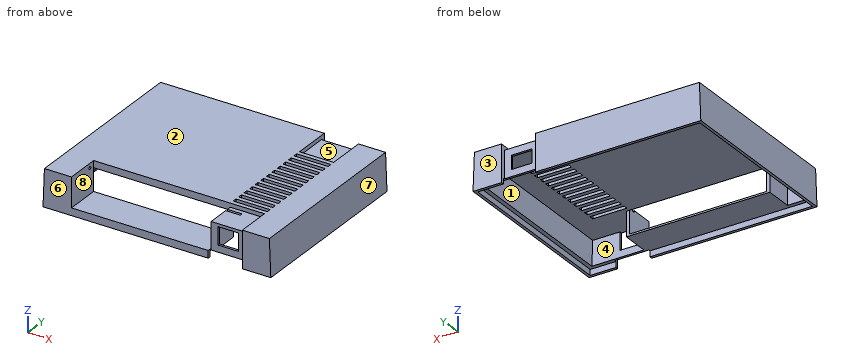
from build123d import *

# Parameters (mm, degrees)
F0_W      = 80
F0_H      = 63
F0_W_2    = 78
F0_H_2    = 61
F1_DEPTH  = 13
F3_DEPTH  = 63
F4_T      = -2.4
F5_DEPTH  = 2
F6_DEPTH  = 1.6
F7_W      = 7.2
F7_H      = 6.2
F8_DEPTH  = 2
F9_W      = 12
F9_H      = 12
F9_H_2    = 10.4
F10_DEPTH = 1.4
F9_H_3    = 1.5
F11_DEPTH = 3
F12_W     = 12
F12_H     = 11.6
F13_DEPTH = 1.6
F14_W     = 7.2
F14_H     = 4.8
F15_DEPTH = 3
F2_W      = 48
F2_H      = 10.4
F16_DEPTH = 12
F17_W     = 1.2
F17_H     = 9.6
F18_DEPTH = 8.6
F19_W     = 9.6
F19_H     = 0.6
F20_DEPTH = 48
F21_D     = 1
F21_DEPTH = 5
F21_TIP   = 0.3004303095
F23_D     = 1
F23_DEPTH = 5
F23_TIP   = 0.3004303095


with BuildPart() as f1:
    # F0 (on Top) → F1 (new body)
    with BuildSketch(Plane.XY):
        Rectangle(F0_W, F0_H)
        Rectangle(F0_W_2, F0_H_2, mode=Mode.SUBTRACT)
        Rectangle(F0_W_2, F0_H_2)
    extrude(amount=F1_DEPTH)

    # F2 (on face) → F3 (cut)
    with BuildSketch(Plane.XZ.offset(31.5)):
        Polygon((-39.5, 13), (-40, 13), (-40, 0), align=None)
        Polygon((39.5, 13), (40, 0), (40, 13), align=None)
    extrude(amount=-F3_DEPTH, mode=Mode.SUBTRACT)

    # F4
    f4_openings = [f1.faces().sort_by_distance(p)[0] for p in [
        (0, 0, 0),
    ]]
    offset(amount=F4_T, openings=f4_openings)

    # F0 (on Top) → F5 (cut)
    with BuildSketch(Plane.XY):
        Rectangle(F0_W_2, F0_H_2)
    extrude(amount=F5_DEPTH, mode=Mode.SUBTRACT)

    # F2 (on face) → F6 (cut)
    with BuildSketch(Plane.XZ.offset(31.5)):
        Polygon((18, 2.6), (18, 0), (30, 0), (30, 13), (18, 13), align=None)
    extrude(amount=-F6_DEPTH, mode=Mode.SUBTRACT)

    # F7 (on face) → F8 (cut)
    with BuildSketch(Plane.XZ.offset(29.9)):
        with Locations((24, 7.5)):
            Rectangle(F7_W, F7_H)
    extrude(amount=-F8_DEPTH, mode=Mode.SUBTRACT)

    # F9 (on face) → F10 (cut)
    with BuildSketch(Plane.XY.offset(13)):
        with Locations((24, 25.5)):
            Rectangle(F9_W, F9_H)
        with Locations((24, -24.7)):
            Rectangle(F9_W, F9_H_2)
    extrude(amount=-F10_DEPTH, mode=Mode.SUBTRACT)

    # F9 (on face) → F11 (cut)
    with BuildSketch(Plane.XY.offset(13)):
        with Locations((24, -17.25)):
            Rectangle(F9_W, F9_H_3)
        with Locations((24, -14.25)):
            Rectangle(F9_W, F9_H_3)
        with Locations((24, -11.25)):
            Rectangle(F9_W, F9_H_3)
        with Locations((24, -8.25)):
            Rectangle(F9_W, F9_H_3)
        with Locations((24, -5.25)):
            Rectangle(F9_W, F9_H_3)
        with Locations((24, 0.75)):
            Rectangle(F9_W, F9_H_3)
        with Locations((24, -2.25)):
            Rectangle(F9_W, F9_H_3)
        with Locations((24, 3.75)):
            Rectangle(F9_W, F9_H_3)
        with Locations((24, 6.75)):
            Rectangle(F9_W, F9_H_3)
        with Locations((24, 9.75)):
            Rectangle(F9_W, F9_H_3)
        with Locations((24, 12.75)):
            Rectangle(F9_W, F9_H_3)
        with Locations((24, 15.75)):
            Rectangle(F9_W, F9_H_3)
        with Locations((24, 18.75)):
            Rectangle(F9_W, F9_H_3)
    extrude(amount=-F11_DEPTH, mode=Mode.SUBTRACT)

    # F12 (on face) → F13 (cut)
    with BuildSketch(Plane(origin=(0, 31.5, 0), x_dir=(-1, 0, 0), z_dir=(0, 1, 0))):
        with Locations((-24, 5.8)):
            Rectangle(F12_W, F12_H)
    extrude(amount=-F13_DEPTH, mode=Mode.SUBTRACT)

    # F14 (on face) → F15 (cut)
    with BuildSketch(Plane(origin=(0, 29.9, 0), x_dir=(-1, 0, 0), z_dir=(0, 1, 0))):
        with Locations((-24, 6.8)):
            Rectangle(F14_W, F14_H)
    extrude(amount=-F15_DEPTH, mode=Mode.SUBTRACT)

    # F2 (on face) → F16 (cut)
    with BuildSketch(Plane.XZ.offset(31.5)):
        with Locations((-6, 7.8)):
            Rectangle(F2_W, F2_H)
    extrude(amount=-F16_DEPTH, mode=Mode.SUBTRACT)

    # F17 (on face) → F18 (join)
    with BuildSketch(Plane(origin=(0, 0, 10.6), x_dir=(1, 0, 0), z_dir=(0, 0, -1))):
        with Locations((18.6, 24.3)):
            Rectangle(F17_W, F17_H)
        with Locations((-30.6, 24.3)):
            Rectangle(F17_W, F17_H)
    extrude(amount=F18_DEPTH)

    # F19 (on face) → F20 (join)
    with BuildSketch(Plane.YZ.offset(-30)):
        with Locations((-24.3, 2.3)):
            Rectangle(F19_W, F19_H)
    extrude(amount=F20_DEPTH)

    # F21 (one way)
    with BuildSketch(Plane.YZ.offset(-30)):
        with Locations((-21.5, 11.4)):
            Circle(F21_D / 2)
    extrude(amount=-F21_DEPTH, mode=Mode.SUBTRACT)
    with Locations(Plane.YZ.offset(-30)):
        with Locations((-21.5, 11.4)):
            with Locations((0, 0, -(F21_DEPTH + F21_TIP / 2))):  # 118° drill point
                Cone(0, F21_D / 2, F21_TIP, mode=Mode.SUBTRACT)

    # F23 (one way)
    with BuildSketch(Plane(origin=(18, 0, 0), x_dir=(0, -1, 0), z_dir=(-1, 0, 0))):
        with Locations((21.5, 11.4)):
            Circle(F23_D / 2)
    extrude(amount=-F23_DEPTH, mode=Mode.SUBTRACT)
    with Locations(Plane(origin=(18, 0, 0), x_dir=(0, -1, 0), z_dir=(-1, 0, 0))):
        with Locations((21.5, 11.4)):
            with Locations((0, 0, -(F23_DEPTH + F23_TIP / 2))):  # 118° drill point
                Cone(0, F23_D / 2, F23_TIP, mode=Mode.SUBTRACT)


solid = f1.part
Input: part model. Units: mm. Frame: model coordinates. Face numbers are marked on the shaded views. A direction names the side the tool comes from. Coordinates: 2 decimals unless noted, no trailing zeros. Loops run counter-clockwise (first coordinate to the right, second up) from the corner with the lowest first, then second, coordinate; pieces in that order, holes last.
(1) Section B-B on z = 7.25. Count the separate pieces of the cut face and the enclosed holes in it, then the cut area to 3 significant figures.
(2) Material intervals for probe 1 along Y at (x, z) = (19.5, 10); probe 2 along Y at (x, z) = (-31, 9.75); probe 3 along Y at (x, z) = (-25.5, 9.5), sorted ascending.
(3) Set-up query: the marked faces 4, 5, 6, 7 and 8. Return all of +Z, -Z, +X, -X, +Y, -Y with unobstructed straight access to the full face (end or side cutting, diameter ignored); none if empty.
(4) Pull-direction query (Y, two-part tool) for the marked faces 1, 2 and 3; classes: released by +Y, released by -Y, zero draft, split by the parting line, or undercut.
(5) First-contact query: pin 1 Ø1.9 at (x, z) = (24, 12) entering from -Y; pin 2 Ø1 at (y, z) = (-8, 10.5) entering from +X; pin 3 Ø2.5 at (y, z) = (-24.5, 5) entering from -X. Flat tips, straight axial feed; report the tip coordinate or a pass-through.
(6) Section C-C on y = 22.5. Return the cut outline in (x, z), then the cut area to 3 significant figures.
(7) Section A-A on x = -17.5. Return the cut outline in (y, z).
Data:
1. separate pieces: 3
1. enclosed holes: 0
1. area: 519 mm2
2. probe 1: y = -29.9 to -29.1, 29.1 to 29.9
2. probe 2: y = -31.5 to -19.5, 29.1 to 31.5
2. probe 3: y = 29.1 to 31.5
3. face 4: -Z
3. face 5: +Z, +Y
3. face 6: +Z, -Z, +X, -X, -Y
3. face 7: +Z, +X, +Y, -Y
3. face 8: +Z, -Y
4. face 1: undercut
4. face 2: zero draft
4. face 3: released by +Y
5. pin 1: stops at y = -29.9
5. pin 2: stops at x = 39.62
5. pin 3: stops at x = -39.86
6. outline: (-40, 0) - (-39, 0) - (-39, 2) - (-37.52, 2) - (-37.19, 10.6) - (37.19, 10.6) - (37.52, 2) - (39, 2) - (39, 0) - (40, 0) - (39.5, 13) - (30, 13) - (30, 11.6) - (18, 11.6) - (18, 13) - (-39.5, 13) - close
6. area: 218 mm2
7. outline: (-31.5, 0) - (-30.5, 0) - (-30.5, 2) - (-19.5, 2) - (-19.5, 2.6) - (-31.5, 2.6) - close; (-19.5, 10.6) - (29.1, 10.6) - (29.1, 2) - (30.5, 2) - (30.5, 0) - (31.5, 0) - (31.5, 13) - (-19.5, 13) - close
